from build123d import *

# Parameters (mm, degrees)
SKETCH1_W           = 85
SKETCH1_H           = 230
SKETCH1_R           = 2.1
BOSS_EXTRUDE2_DEPTH = 13
FILLET1_R           = 5
FILLET2_R           = 5
CUT_EXTRUDE2_DEPTH  = 35
CUT_EXTRUDE3_DEPTH  = 14
SKETCH6_R           = 1.55
CUT_EXTRUDE4_DEPTH  = 7
SKETCH9_W           = 25
SKETCH9_H           = 110
CUT_EXTRUDE5_DEPTH  = 8
SKETCH13_R          = 5
SKETCH13_W          = 10
SKETCH13_H          = 230
BOSS_EXTRUDE4_DEPTH = 7
SKETCH14_W          = 15
SKETCH14_H          = 41
CUT_EXTRUDE6_DEPTH  = 6.5
SKETCH16_R          = 4.5
CUT_EXTRUDE8_DEPTH  = 25
SKETCH20_W          = 10
SKETCH20_H          = 27
CUT_EXTRUDE9_DEPTH  = 7


with BuildPart() as part:
    # Sketch1 → Boss-Extrude2 (new body)
    with BuildSketch(Plane.XY):
        with Locations((42.5, 115)):
            Rectangle(SKETCH1_W, SKETCH1_H)
        with Locations(Location((77.7, 181.8, 0), (0, 0, 180))):
            Circle(SKETCH1_R, mode=Mode.SUBTRACT)
        with Locations(Location((77.7, 154.8, 0), (0, 0, 180))):
            Circle(SKETCH1_R, mode=Mode.SUBTRACT)
        with Locations(Location((77.7, 75.2, 0), (0, 0, 180))):
            Circle(SKETCH1_R, mode=Mode.SUBTRACT)
        with Locations(Location((77.7, 48.2, 0), (0, 0, 180))):
            Circle(SKETCH1_R, mode=Mode.SUBTRACT)
    extrude(amount=BOSS_EXTRUDE2_DEPTH)

    # Fillet1
    fillet1_edges = [part.edges().sort_by_distance(p)[0] for p in [
        (85, 230, 6.5),
        (85, 0, 6.5),
    ]]
    fillet(fillet1_edges, radius=FILLET1_R)

    # Fillet2
    fillet2_edges = [part.edges().sort_by_distance(p)[0] for p in [
        (85, 115, 13),
        (40, 230, 13),
        (83.535533906, 228.535533906, 13),
        (83.535533906, 1.464466094, 13),
        (40, 0, 13),
    ]]
    fillet(fillet2_edges, radius=FILLET2_R)

    # Sketch5 → Cut-Extrude2 (cut)
    with BuildSketch(Plane.ZY):
        with BuildLine():
            Line((6.5, 119.5), (0, 119.5))
            Line((0, 119.5), (0, 110.5))
            Line((0, 110.5), (6.5, 110.5))
            ThreePointArc((6.5, 110.5), (11, 115), (6.5, 119.5))
        make_face()
        with BuildLine():
            Line((0, 146.5), (6.5, 146.5))
            ThreePointArc((6.5, 146.5), (11, 151), (6.5, 155.5))
            Line((6.5, 155.5), (0, 155.5))
            Line((0, 155.5), (0, 146.5))
        make_face()
        with BuildLine():
            Line((0, 83.5), (0, 74.5))
            Line((0, 74.5), (6.5, 74.5))
            ThreePointArc((6.5, 74.5), (11, 79), (6.5, 83.5))
            Line((6.5, 83.5), (0, 83.5))
        make_face()
    extrude(amount=-CUT_EXTRUDE2_DEPTH, mode=Mode.SUBTRACT)

    # Sketch4 → Cut-Extrude3 (cut)
    with BuildSketch(Plane.XY.offset(13)):
        with BuildLine():
            Line((27, 119.5), (7, 119.5))
            Line((7, 119.5), (7, 110.5))
            Line((7, 110.5), (27, 110.5))
            ThreePointArc((27, 110.5), (28.767766953, 111.232233047), (29.5, 113))
            Line((29.5, 113), (29.5, 117))
            ThreePointArc((29.5, 117), (28.767766953, 118.767766953), (27, 119.5))
        make_face()
        with BuildLine():
            ThreePointArc((4, 117.5), (4.585786438, 118.914213562), (6, 119.5))
            Line((6, 119.5), (7, 119.5))
            Line((7, 119.5), (7, 110.5))
            Line((7, 110.5), (6, 110.5))
            ThreePointArc((6, 110.5), (4.585786438, 111.085786438), (4, 112.5))
            Line((4, 112.5), (4, 117.5))
        make_face()
        with BuildLine():
            ThreePointArc((29.5, 153), (28.767766953, 154.767766953), (27, 155.5))
            Line((27, 155.5), (7, 155.5))
            Line((7, 155.5), (6, 155.5))
            ThreePointArc((6, 155.5), (4.585786438, 154.914213562), (4, 153.5))
            Line((4, 153.5), (4, 148.5))
            ThreePointArc((4, 148.5), (4.585786438, 147.085786438), (6, 146.5))
            Line((6, 146.5), (7, 146.5))
            Line((7, 146.5), (27, 146.5))
            ThreePointArc((27, 146.5), (28.767766953, 147.232233047), (29.5, 149))
            Line((29.5, 149), (29.5, 153))
        make_face()
        with BuildLine():
            Line((7, 74.5), (27, 74.5))
            ThreePointArc((27, 74.5), (28.767766953, 75.232233047), (29.5, 77))
            Line((29.5, 77), (29.5, 81))
            ThreePointArc((29.5, 81), (28.767766953, 82.767766953), (27, 83.5))
            Line((27, 83.5), (7, 83.5))
            Line((7, 83.5), (6, 83.5))
            ThreePointArc((6, 83.5), (4.585786438, 82.914213562), (4, 81.5))
            Line((4, 81.5), (4, 76.5))
            ThreePointArc((4, 76.5), (4.585786438, 75.085786438), (6, 74.5))
            Line((6, 74.5), (7, 74.5))
        make_face()
    extrude(amount=-CUT_EXTRUDE3_DEPTH, mode=Mode.SUBTRACT)

    # Sketch6 → Cut-Extrude4 (cut)
    with BuildSketch(Plane(origin=(0, 0, 0), x_dir=(-1, 0, 0), z_dir=(0, 0, -1))):
        with Locations((-12, 107.9)):
            Circle(SKETCH6_R)
        with Locations((-4, 107.9)):
            Circle(SKETCH6_R)
        with Locations((-12, 122.1)):
            Circle(SKETCH6_R)
        with Locations(Location((-4, 122.1, 0), (0, 0, 180))):
            Circle(SKETCH6_R)
        with Locations(Location((-12, 158.1, 0), (0, 0, 180))):
            Circle(SKETCH6_R)
        with Locations((-12, 143.9)):
            Circle(SKETCH6_R)
        with Locations((-4, 143.9)):
            Circle(SKETCH6_R)
        with Locations(Location((-4, 158.1, 0), (0, 0, 180))):
            Circle(SKETCH6_R)
        with Locations(Location((-12, 86.1, 0), (0, 0, 180))):
            Circle(SKETCH6_R)
        with Locations(Location((-4, 86.1, 0), (0, 0, 180))):
            Circle(SKETCH6_R)
        with Locations((-4, 71.9)):
            Circle(SKETCH6_R)
        with Locations((-12, 71.9)):
            Circle(SKETCH6_R)
    extrude(amount=-CUT_EXTRUDE4_DEPTH, mode=Mode.SUBTRACT)

    # Sketch9 → Cut-Extrude5 (cut)
    with BuildSketch(Plane(origin=(0, 0, 0), x_dir=(-1, 0, 0), z_dir=(0, 0, -1))):
        Polygon((0, 170), (0, 230), (-70, 230), (-70, 170), (-45, 170), align=None)
        with Locations((-57.5, 115)):
            Rectangle(SKETCH9_W, SKETCH9_H)
        Polygon((-45, 60), (-70, 60), (-70, 0), (0, 0), (0, 60), align=None)
    extrude(amount=-CUT_EXTRUDE5_DEPTH, mode=Mode.SUBTRACT)

    # Sketch13 → Boss-Extrude4 (add)
    with BuildSketch(Plane(origin=(0, 0, 8), x_dir=(-1, 0, 0), z_dir=(0, 0, -1))):
        with Locations((-10, 15)):
            Circle(SKETCH13_R)
        with Locations((-40, 115)):
            Rectangle(SKETCH13_W, SKETCH13_H)
    extrude(amount=BOSS_EXTRUDE4_DEPTH)

    # Sketch14 → Cut-Extrude6 (cut)
    with BuildSketch(Plane(origin=(0, 0, 0), x_dir=(-1, 0, 0), z_dir=(0, 0, -1))):
        with Locations((-77.5, 168.3)):
            Rectangle(SKETCH14_W, SKETCH14_H)
        with Locations((-77.5, 61.7)):
            Rectangle(SKETCH14_W, SKETCH14_H)
    extrude(amount=-CUT_EXTRUDE6_DEPTH, mode=Mode.SUBTRACT)

    # Sketch16 → Cut-Extrude8 (cut)
    with BuildSketch(Plane.ZY.offset(-35)):
        with Locations(Location((6.5, 115, 0), (0, 0, 333.612200039))):
            Circle(SKETCH16_R)
        with Locations(Location((6.5, 151, 0), (0, 0, 333.612200039))):
            Circle(SKETCH16_R)
        with Locations(Location((6.5, 79, 0), (0, 0, 333.612200039))):
            Circle(SKETCH16_R)
    extrude(amount=-CUT_EXTRUDE8_DEPTH, mode=Mode.SUBTRACT)

    # Sketch20 → Cut-Extrude9 (cut)
    with BuildSketch(Plane(origin=(0, 0, 1), x_dir=(-1, 0, 0), z_dir=(0, 0, -1))):
        with Locations((-40, 25.5)):
            Rectangle(SKETCH20_W, SKETCH20_H)
    extrude(amount=-CUT_EXTRUDE9_DEPTH, mode=Mode.SUBTRACT)


solid = part.part
Work out the finished part from the listing and answer in its coordinate system (mm). A direction names the side the tool comes from. Round coordinates to 2 decimals unless told otherwise and drop trailing zeros. Order: outer loops, then holes, each group sorted by start corner. A loop starts at its lowest first (then second) coordinate and runs counter-clockwise, first axis right, second up. Notation, with made-up numbers: M 68.25,22.5 L 81.25,22.5 A22 ccw 81.25,48.5 Z; hole C 48.25,-28.75 d10. An arc over 180 degrees is marked long. Put each result on its own line as item: value. Start each with the question number.
Q1. Section C-C, the plane y = 48.2 is taken. Write down the section's boundary in (x, z).
Q2. Flat-ended cylindrical pins translate along their axes: pin 1 (5 mm diameter, centred on y = 52, z = 3, fed in from +X); pin 2 (0.9 mm diameter, centred on x = 4.5, y = 86, fed in from -Z); pin 3 (7 mm diameter, centred on y = 79.5, z = 3, fed in from -X); pin 4 (6 mm diameter, centred on x = 48.5, z = 2, fed in from -Y). Find the tip coordinate at first contact, or state that the pin passes through.
Q3. Section D-D, the plane y = 15 is taken. Write down the section's boundary in (x, z), and give its area (3 significant figures).
Q4. A tool of negligible diameter and unlimited length cuts with its end or side. For faces 1 (the flat face through (17, 155.5, 5)), 2 (the flat face through (78, 169, 6.5)), 3 (the flat face through (40, 200, 1)), 4 (the flat face through (10, 15, 1)), 5 (the cylindrical face through (43.269, 149.288, 10.662)), from which of +Z, -Z, +X, -X, +Y, -Y can it reach the whole face along a straight path? Write none if from no direction.
Q5. Section A-A, the plane x = 23 is taken. Write down the section's boundary in (y, z).
Q6. For a pull along Y with two mould halves and no side action, classify faces 6 (the cylindrical face through (39, 228, 12)), 7 (the flat face through (17, 146.5, 5)), 8 (the flat face through (75, 0, 4)), 9 (the flat face through (45, 133, 4)) as pulls with the +Y half, pulls with the -Y half, needs draft (parallel to the pull), parting line crosses it, or undercut.
Q7. Section B-B, the plane y = 115 is taken. Write down the section's boundary in (x, z), and give its area (3 significant figures).
Q8. Straight lines are drawn through the part: L1, parallel to Y at x = 23, z = 6; L2, parallel to X at y = 158.1, z = 4.75; L3, parallel to Y at x = 10, z = 5.25. For each, find the intervals that lie inside material, in ascending order. Write a range as [from, to].
Findings below:
1. outline: M 0,8 L 35,8 L 35,1 L 45,1 L 45,8 L 70,8 L 70,6.5 L 75.6,6.5 L 75.6,13 L 0,13 Z; M 79.8,6.5 L 85,6.5 L 85,8 A5 ccw 80,13 L 79.8,13 Z
2. pin 1: stops at x = 45
2. pin 2: stops at z = 7
2. pin 3: stops at x = 35
2. pin 4: passes through
3. outline: M 0,8 L 5,8 L 5,1 L 15,1 L 15,8 L 70,8 L 70,0 L 85,0 L 85,8 A5 ccw 80,13 L 0,13 Z
3. area: 610 mm^2
4. face 1: -Z
4. face 2: -Z, +X
4. face 3: -Z, -X, +Y
4. face 4: -Z, -X, -Y
4. face 5: -X
5. outline: M 0,8 L 60,8 L 60,0 L 74.5,0 L 74.5,13 L 5,13 A5 ccw Z; M 83.5,0 L 110.5,0 L 110.5,13 L 83.5,13 Z; M 119.5,0 L 146.5,0 L 146.5,13 L 119.5,13 Z; M 155.5,0 L 170,0 L 170,8 L 230,8 A5 ccw 225,13 L 155.5,13 Z
6. face 6: pulls with the +Y half
6. face 7: undercut
6. face 8: pulls with the -Y half
6. face 9: needs draft
7. outline: M 0,11 L 4,11 L 4,13 L 0,13 Z; M 29.5,11 L 60,11 L 60,8 L 70,8 L 70,0 L 85,0 L 85,8 A5 ccw 80,13 L 29.5,13 Z; M 35,0 L 45,0 L 45,2 L 35,2 Z
7. area: 329 mm^2
8. L1: y = [60, 74.5], [83.5, 110.5], [119.5, 146.5], [155.5, 170]
8. L2: x = [0, 2.45], [5.55, 10.45], [13.55, 45]
8. L3: y = [10, 20], [60, 74.5], [83.5, 110.5], [119.5, 146.5], [155.5, 170]
